Check sheet for the modelled part. Datum: model origin and axes. Units: mm. A direction names the side the tool comes from. Give positions to 0.01 mm unless a question says otherwise; leave off trailing zeros. Order: outer loops, then holes, each group sorted by start corner. A loop starts at its lowest first (then second) coordinate and runs counter-clockwise, first axis right, second up. Notation, with made-up numbers: (33.25, 19.25) - (39.25, 19.25) arc R13 cw to (39.25, 34.25) - close; hole circle Ø8 at (53, 76). An arc over 180 degrees is marked (long way). Answer in a Markdown table with one row per item.
Autodesk Inventor part; units mm, degrees
ref_plane "Arbeitsebene1" through (26.5, 0, 0) normal (1, 0, 0) x (0, 0, -1)
ref_plane "YZ Plane" through (0, 0, 0) normal (1, 0, 0) x (0, 1, 0)
ref_plane "XZ Plane" through (0, 0, 0) normal (0, 1, 0) x (-1, 0, 0)
sketch "Skizze1" plane through (0, 0, 0) normal (1, 0, 0) x (0, 1, 0)
  line L0 (0, 0) -> (0, -100)
  line L1 (0, -100) -> (41.1159, -51)
  line L2 (0, 0) -> (41.1159, -49)
  circle A0 centre (44.47, -50) radius 3.5
  circle A1 centre (44.47, -50) radius 1.75
  dimension "d0" = 40
  dimension "d1" = 3.5
  dimension "d2" = 7
  dimension "d3" = 2
  dimension "d4" = 100
extrude "Extrusion1" add sketch "Skizze1" along normal blind 28.5
sketch "Skizze2" plane through (0, 0, -100) normal (0, -1, 0) x (1, 0, 0)
  line L0 (0, 100) -> (0, 0)
  line L1 (0, 0) -> (28.5, 0)
  line L2 (28.5, 100) -> (28.5, 0)
  line L3 (0, 100) -> (28.5, 100)
extrude "Extrusion2" add sketch "Skizze2" along normal blind 5
sketch "Skizze3" plane through (28.5, 0, 0) normal (1, 0, 0) x (0, 0, -1)
  line L0 (100, 0) -> (51, 41.1159)
  arc A0 (51, 41.1159) -> (49, 41.1159) centre (50, 44.47) ccw
  line L1 (49, 41.1159) -> (0, 0)
  line L2 (0, 0) -> (0, -5)
  line L3 (100, -5) -> (0, -5)
  line L4 (100, 0) -> (100, -5)
  circle A1 centre (50, 44.47) radius 1.75
  line L5 (49, 41.1159) -> (0, 0)
  line L6 (0, 0) -> (100, 0)
  line L7 (0, 0) -> (0, -5)
  line L8 (0, -2.5) -> (100, -2.5)
extrude "Extrusion3" cut sketch "Skizze3" against normal blind 24 contours L4 L8 L2 L6
sketch "Skizze4" plane through (28.5, 0, 0) normal (1, 0, 0) x (0, 0, -1)
  line L0 (0, 0) -> (100, 0)
  line L1 (100, -5) -> (0, -5)
  line L2 (0, 0) -> (13.75, 0)
  line L3 (13.75, 0) -> (13.75, -5)
  line L4 (13.75, -5) -> (0, -5)
  line L5 (0, -5) -> (0, 0)
  line L6 (100, 0) -> (51, 41.1159)
  line L7 (100, 0) -> (86.25, 0)
  line L8 (86.25, 0) -> (86.25, -5)
  line L9 (86.25, -5) -> (100, -5)
  line L10 (100, -5) -> (100, 0)
  dimension "d11" = 72.5
extrude "Extrusion4" cut sketch "Skizze4" against normal through all contours L0 L3 L1 L5 | L0 L10 L1 L8
sketch "Skizze5" plane through (28.5, 0, 0) normal (1, 0, 0) x (0, 0, -1)
  line L0 (86.25, -5) -> (86.25, -2.5)
  line L1 (86.25, -2.5) -> (13.75, -2.5)
  line L2 (13.75, -2.5) -> (13.75, -5)
  line L3 (86.25, -5) -> (13.75, -5)
  point P0 (0, 0)
extrude "Extrusion5" cut sketch "Skizze5" against normal blind 14.5
ref_plane "Arbeitsebene1" through (26.5, 0, 0) normal (1, 0, 0) x (0, 0, -1)
sketch "Skizze6" plane through (26.5, 0, 0) normal (1, 0, 0) x (0, 0, -1)
  line L0 (49, 41.1159) -> (0, 0)
  line L1 (100, 0) -> (51, 41.1159)
  line L2 (13.75, 0) -> (0, 0)
  line L3 (13.75, 0) -> (86.25, 0)
  line L4 (100, 0) -> (86.25, 0)
  line L5 (3.1114, 0) -> (50, 39.3442)
  line L6 (50, 39.3442) -> (96.8886, 0)
  circle A0 centre (50, 44.47) radius 1.75
  dimension "d17" = 2
extrude "Extrusion6" cut sketch "Skizze6" against normal blind 3.5 contours L2 L5 L6 L4 L3
sketch "Skizze7" plane through (23, 0, 0) normal (1, 0, 0) x (0, 0, -1)
  line L0 (96.8886, 0) -> (3.1114, 0)
  line L1 (50, 39.3442) -> (96.8886, 0)
  line L2 (3.1114, 0) -> (50, 39.3442)
  line L3 (96.8886, 0) -> (3.1114, 0)
  line L4 (6.2229, 0) -> (50, 36.7334)
  line L5 (50, 36.7334) -> (93.7771, 0)
  line L6 (100, 0) -> (86.25, 0)
  point P0 (0, 0)
  dimension "d20" = 2
extrude "Extrusion7" cut sketch "Skizze7" along normal through all contours L0 L4 L5
sketch "Skizze8" plane through (0, 0, 0) normal (-1, 0, 0) x (0, 0, 1)
  line L0 (-100, 0) -> (-86.25, 0)
  line L1 (-13.75, 0) -> (0, 0)
  line L2 (-13.75, 0) -> (-86.25, 0)
  line L3 (-49, 41.1159) -> (0, 0)
  line L4 (-100, 0) -> (-51, 41.1159)
  circle A0 centre (-50, 44.47) radius 1.75
  line L5 (-93.7771, 0) -> (-96.8886, 0)
  line L6 (-50, 39.3442) -> (-96.8886, 0)
  line L7 (-92.1215, 4) -> (-7.8785, 4)
  line L8 (-3.1114, 0) -> (-50, 39.3442)
  line L9 (-93.7771, 0) -> (-50, 36.7334)
  line L10 (-50, 36.7334) -> (-6.2229, 0)
  point P0 (-10.9899, 4)
  point P1 (-89.0101, 4)
  dimension "d23" = 4
extrude "Extrusion8" cut sketch "Skizze8" against normal up to surface (23 mm away) contours L9 L10 L7
properties part number "roof_foot"
(1) Access from +Z, -Z, +X, -X, +Y, -Y to the whole of each face (thin tool, end or side, straight path). Record for faces 1 (the flat face through (11, 4, -51)), 2 (the flat face through (14, -4, -49)), 3 (the flat face through (9, -2.5, -49)), 4 (the flat face through (24.77, 19.4, -26.23)), 5 (the flat face through (6, -3, -13.75)).
Geometry says:
| item | result |
|---|---|
| face 1 | +X, -X |
| face 2 | +Z, -Z, +X, -Y |
| face 3 | +Z, -Z, +X |
| face 4 | -Y |
| face 5 | +Z, +X, -X, -Y |
(2) Gauge pin test, flat ends, axial feed: P1, Ø3, axis at x = 17, z = -65, coming from the -Y side; P2, Ø4, axis at x = 19, y = 9, coming from the +Z side; P3, Ø8, axis at x = 24, z = -22.5, coming from the +Y side. Record the tip position at first contact, or that the pin passes through.
Geometry says:
| item | result |
|---|---|
| P1 | y = 0 |
| P2 | z = -8.34 |
| P3 | y = 22.24 |
(3) Mould release check, pull along X, two halves, no side actions. Record for faces 6 (the flat face through (26.5, 29, -60)), 7 (the flat face through (0, 2, -50)), 8 (the flat face through (11, 0, -49)), 9 (the flat face through (4.5, -1, -49)): pulls with the +X half, pulls with the -X half, needs draft (parallel to the pull), parting line crosses it, or undercut.
Geometry says:
| item | result |
|---|---|
| face 6 | undercut |
| face 7 | pulls with the -X half |
| face 8 | needs draft |
| face 9 | pulls with the +X half |
(4) Cross-section at B-B, the plane y = 44.47. Record the cut outline in (x, z), then the cut area to 4 significant figures.
Geometry says:
| item | result |
|---|---|
| outline | (0, -53.5) - (28.5, -53.5) - (28.5, -51.75) - (0, -51.75) - close; (0, -48.25) - (28.5, -48.25) - (28.5, -46.5) - (0, -46.5) - close |
| area | 99.75 mm² |
(5) Cross-section at D-D, the plane x = 19.25. Record the cut outline in (y, z).
Geometry says:
| item | result |
|---|---|
| outline | (0, -100) - (41.12, -51) arc R3.5 ccw (long way) to (41.12, -49) - (0, 0) - close; hole (4, -89.01) - (36.73, -50) - (4, -10.99) - close; hole circle Ø3.5 at (44.47, -50) |
(6) Cross-section at C-C, the plane z = -20.5. Record the cut outline in (x, y).
Geometry says:
| item | result |
|---|---|
| outline | (0, -5) - (14, -5) - (14, -2.5) - (4.5, -2.5) - (4.5, 0) - (23, 0) - (23, 4) - (0, 4) - close; (0, 11.98) - (23, 11.98) - (23, 14.59) - (26.5, 14.59) - (26.5, 11.98) - (28.5, 11.98) - (28.5, 17.2) - (0, 17.2) - close |
(7) Thickness scan on L1, parallel to Z at x = 14.5, y = 44.47; L2, parallel to Y at x = 7.5, z = -84; L3, parallel to Y at x = 9.5, z = -35.5. Record the ranges inside material, lowest first.
Geometry says:
| item | result |
|---|---|
| L1 | -53.5 to -51.75, -48.25 to -46.5 |
| L2 | -5 to -2.5, 0 to 4, 8.2 to 13.43 |
| L3 | -5 to -2.5, 0 to 4, 24.57 to 29.79 |
(8) Cross-section at A-A, the plane x = 11.25. Record the cut outline in (y, z), then the cut area to 3 significant figures.
Geometry says:
| item | result |
|---|---|
| outline | (-5, -86.25) - (-2.5, -86.25) - (-2.5, -13.75) - (-5, -13.75) - close; (0, -100) - (41.12, -51) arc R3.5 ccw (long way) to (41.12, -49) - (0, 0) - close; hole (4, -89.01) - (36.73, -50) - (4, -10.99) - close; hole circle Ø3.5 at (44.47, -50) |
| area | 1,030 mm² |
